Build history of the part. All positions in model axes, mm. A direction names the side the tool comes from. Round coordinates to 2 decimals unless told otherwise and drop trailing zeros. Loops run counter-clockwise (first coordinate to the right, second up) from the corner with the lowest first, then second, coordinate; pieces in that order, holes last. Notation, with made-up numbers: M 61.25,1 L 67.25,1 A20 ccw 67.25,17 Z; hole C 45,76 d8. An arc over 180 degrees is marked long. One line per item, written item: value.
```python
from build123d import *

# Parameters (mm, degrees)
F0_W     = 38.1
F0_H     = 50.8
F1_DEPTH = 762
F3_DEPTH = 38.1
F5_DEPTH = 25.4


with BuildPart() as f1:
    # F0 (on Right) → F1 (new body)
    with BuildSketch(Plane.YZ):
        with Locations((19.05, 25.4)):
            Rectangle(F0_W, F0_H)
    extrude(amount=F1_DEPTH)

    # F2 (on face) → F3 (cut)
    with BuildSketch(Plane.XY.offset(50.8)):
        with BuildLine():
            ThreePointArc((6.35, -2.54), (19.05, -15.24), (31.75, -2.54))
            ThreePointArc((31.75, -2.54), (19.05, 10.16), (6.35, -2.54))
        make_face()
        with BuildLine():
            ThreePointArc((57.15, -2.54), (69.85, -15.24), (82.55, -2.54))
            ThreePointArc((82.55, -2.54), (69.85, 10.16), (57.15, -2.54))
        make_face()
        with BuildLine():
            ThreePointArc((107.95, -2.54), (120.65, -15.24), (133.35, -2.54))
            ThreePointArc((133.35, -2.54), (120.65, 10.16), (107.95, -2.54))
        make_face()
    extrude(amount=-F3_DEPTH, mode=Mode.SUBTRACT)

    # F4 (on face) → F5 (cut)
    with BuildSketch(Plane.XY.offset(50.8)):
        with BuildLine():
            ThreePointArc((31.75, -2.54), (44.45, -15.24), (57.15, -2.54))
            ThreePointArc((57.15, -2.54), (44.45, 10.16), (31.75, -2.54))
        make_face()
        with BuildLine():
            ThreePointArc((158.75, -2.54), (146.05, 10.16), (133.35, -2.54))
            ThreePointArc((133.35, -2.54), (146.05, -15.24), (158.75, -2.54))
        make_face()
        with BuildLine():
            ThreePointArc((107.95, -2.54), (95.25, 10.16), (82.55, -2.54))
            ThreePointArc((82.55, -2.54), (95.25, -15.24), (107.95, -2.54))
        make_face()
    extrude(amount=-F5_DEPTH, mode=Mode.SUBTRACT)


solid = f1.part
```
Item 1: Which spindle directions (+Z, -Z, +X, -X, +Y, -Y) get a long thin tool onto all of the face, cutting with end or side? Do faces 5 (the face through (70.093, 10.158, 32.017)), 6 (the face through (376, 38.1, 25)). Say none if no direction does.
Check values:
face 5: +Z, -Y
face 6: +Z, -Z, +X, -X, +Y
Item 2: Wall check: line 1 along X through (y, z) = (8, 16); line 2 along Y through (x, z) = (87, 29). Give the ranges that are in metal, low to high.
Check values:
line 1: x = 0 to 11.96, 26.14 to 62.76, 76.94 to 113.56, 127.74 to 762
line 2: y = 7.12 to 38.1
Item 3: Pull direction X, two halves, no side cores. Call faces 1 (the face through (0, 19, 26)), 2 (the face through (376, 19, 0)), 3 (the face through (95.493, 10.158, 38.278)), 4 (the face through (120.893, 10.158, 32.017)): pulls with the +X half, pulls with the -X half, needs draft (parallel to the pull), parting line crosses it, or undercut.
Check values:
face 1: pulls with the -X half
face 2: needs draft
face 3: undercut
face 4: undercut
Item 4: Slice it at B-B, the plane x = 98.5. Give the cut face in (y, z).
Check values:
outline: M 0,0 L 38.1,0 L 38.1,50.8 L 9.74,50.8 L 9.74,25.4 L 0,25.4 Z
Item 5: Slice it at A-A, the plane z = 34. Give the cut face in (x, y), and give its area (3 significant figures).
Check values:
outline: M 0,0 L 6.61,0 A12.7 cw 31.49,0 L 32.01,0 A12.7 cw 56.89,0 L 57.41,0 A12.7 cw 82.29,0 L 82.81,0 A12.7 cw 107.69,0 L 108.21,0 A12.7 cw 133.09,0 L 133.61,0 A12.7 cw 158.49,0 L 762,0 L 762,38.1 L 0,38.1 Z
area: 27,900 mm2
Item 6: Drop a flat-ended pin along its axis: P1, Ø5, axis at x = 15, y = 4, coming from the +Z side. Give the stop position or say it passes through.
Check values:
P1: stops at z = 12.7
